```python
from build123d import *

# Parameters (mm, degrees)
F0_R     = 1.1
F0_R_2   = 2.4
F1_DEPTH = 2


with BuildPart() as f1:
    # F0 (on Front) → F1 (new body)
    with BuildSketch(Plane.XZ):
        with BuildLine():
            ThreePointArc((-19.499595, -13.991633), (-23.127131, -6.413721), (-23.920639, 1.950137))
            ThreePointArc((-23.920639, 1.950137), (-24.031346, 2.306574), (-24.358051, 2.487038))
            Line((-24.358051, 2.487038), (-35.282341, 3.828372))
            ThreePointArc((-35.282341, 3.828372), (-35.656626, 3.721729), (-35.841068, 3.37903))
            ThreePointArc((-35.841068, 3.37903), (-34.690696, -9.620582), (-28.981463, -21.355908))
            ThreePointArc((-28.981463, -21.355908), (-28.646861, -21.554664), (-28.271112, -21.453304))
            Line((-28.271112, -21.453304), (-19.598006, -14.677131))
            ThreePointArc((-19.598006, -14.677131), (-19.41091, -14.354178), (-19.499595, -13.991633))
        make_face()
        with Locations((-27.783877, -17.324135)):
            Circle(F0_R, mode=Mode.SUBTRACT)
        with Locations((-30.026085, -12.437212)):
            Circle(F0_R_2, mode=Mode.SUBTRACT)
        with Locations((-23.815699, -13.75)):
            Circle(F0_R_2, mode=Mode.SUBTRACT)
        with Locations((-26.56296, -7.117524)):
            Circle(F0_R_2, mode=Mode.SUBTRACT)
        with Locations((-32.221958, -4.242101)):
            Circle(F0_R_2, mode=Mode.SUBTRACT)
        with Locations((-32.758802, 0.800339)):
            Circle(F0_R, mode=Mode.SUBTRACT)
        with Locations((-27.5, 0)):
            Circle(F0_R_2, mode=Mode.SUBTRACT)
    extrude(amount=F1_DEPTH)


solid = f1.part
```
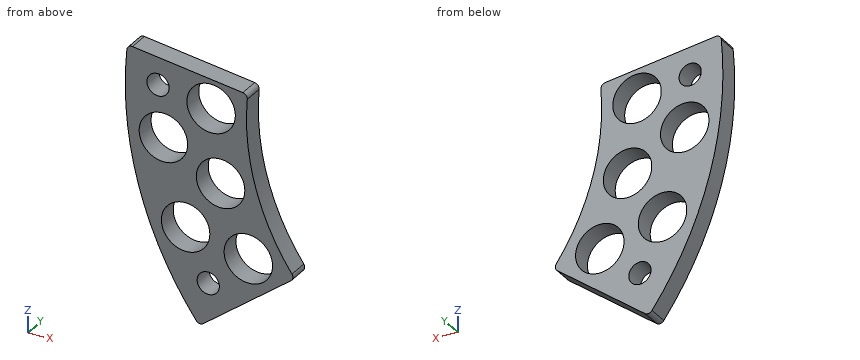
Source: CAD feature listing. Evaluate the final solid. Frame: model axes, mm. Coordinates: 2 decimals unless noted, no trailing zeros. Loops run counter-clockwise (first coordinate to the right, second up) from the corner with the lowest first, then second, coordinate; pieces in that order, holes last. Notation, with made-up numbers: (-40, 13.5) - (2, 13.5) arc R23 cw to (2, 36.5) - close; hole circle Ø6 at (4.5, 38). An arc over 180 degrees is marked (long way). Answer as CSV lines item,"result".
1. Section C-C (z = 0). Return loops of the section in (x, y), then the cut area to 3 significant figures.
Established:
outline,"(-36, -2) - (-33.51, -2) - (-33.51, 0) - (-36, 0) - close; (-32, -2) - (-29.9, -2) - (-29.9, 0) - (-32, 0) - close; (-25.1, -2) - (-24, -2) - (-24, 0) - (-25.1, 0) - close"
area,"11.4 mm2"
2. Section B-B (x = -33.5). Return loops of the section in (y, z).
Established:
outline,"(-2, -13.18) - (0, -13.18) - (0, -6.27) - (-2, -6.27) - close; (-2, -2.21) - (0, -2.21) - (0, -0.01) - (-2, -0.01) - close; (-2, 1.61) - (0, 1.61) - (0, 3.61) - (-2, 3.61) - close"
3. Contact query for a flat-ended pin moving along its axis: pin 1 (4 mm diameter, centred on x = -26.56, z = -7.12, fed in from -Y). Output: stop coordinate, or through.
Established:
pin 1,"passes through"
4. Ray query, line 1 (Z direction, x = -32.75, y = -1.4); line 2 (Z direction, x = -27, y = -1.55); line 3 (X direction, y = -0.4, z = -4.25). Return the intervals inside material, ascending.
Established:
line 1,"z = -14.95 to -6.58, -1.9 to -0.3, 1.9 to 3.52"
line 2,"z = -20.46 to -18.1, -16.55 to -9.48, -4.76 to -2.35, 2.35 to 2.81"
line 3,"x = -35.75 to -34.62, -29.82 to -23.62"
5. Section A-A (z = -8.5). Return loops of the section in (x, y), then the cut area to 3 significant figures.
Established:
outline,"(-34.98, -2) - (-28.52, -2) - (-28.52, 0) - (-34.98, 0) - close; (-24.6, -2) - (-22.44, -2) - (-22.44, 0) - (-24.6, 0) - close"
area,"17.2 mm2"
6. Section D-D (y = -0.65). Return loops of the section in (x, z), then the cut area to 3 significant figures.
Established:
outline,"(-35.84, 3.38) arc R36 ccw to (-28.98, -21.36) arc R0.5 ccw to (-28.27, -21.45) - (-19.6, -14.68) arc R0.5 ccw to (-19.5, -13.99) arc R24 cw to (-23.92, 1.95) arc R0.5 ccw to (-24.36, 2.49) - (-35.28, 3.83) arc R0.5 ccw to start; hole circle Ø4.8 at (-32.22, -4.24); hole circle Ø2.2 at (-32.76, 0.8); hole circle Ø4.8 at (-30.03, -12.44); hole circle Ø4.8 at (-27.5, 0); hole circle Ø4.8 at (-26.56, -7.12); hole circle Ø2.2 at (-27.78, -17.32); hole circle Ø4.8 at (-23.82, -13.75)"
area,"172 mm2"
